Design review of the part built by this model. Coordinates are the model's own, in mm. A direction names the side the tool comes from. Coordinates: 2 decimals unless noted, no trailing zeros. Write each loop counter-clockwise with the first axis right and the second up, starting at its lowest first coordinate (ties: lowest second). Pieces come first, ordered by that corner, then holes.
Q1. For faces 1 (the cylindrical face through (-7.43, 0.76, 15.4)), 2 (the cylindrical face through (12.4, 0.76, 19.43)), list the 3-axis set-ups (+Z, -Z, +X, -X, +Y, -Y) from which the entire face can be reached by the end or side of a thin tool; tool diameter is ignored.
Q2. Take a section at A-A, the plane x = 0. Write out the cut boundary in (y, z), plus the area to 3 significant figures.
Q3. The part is to be moulded in two halves that separate along X. For faces 3 (the flat face through (-3, 1.5, -19)), 4 (the cylindrical face through (7.4, 0.76, 15.43)), 5 (the cylindrical face through (43.4, 0.74, -30.18)), say which applies: released by +X, released by -X, zero draft, split by the parting line, or undercut.
Q4. Take a section at C-C, the plane z = 15. Write out the cut boundary in (x, y).
Q5. Take a section at B-B, the plane x = 24.1. Write out the cut boundary in (y, z), plus the area to 3 significant figures.
Q6. Take a section at D-D, the plane y = 1. State how many separate pieces and enclosed holes the cut face has, plus the area to 3 significant figures.
Q7. For L1, parallel to X at y = 0.45, z = -27; L2, parallel to X at y = 0.65, z = 6.5; L3, parallel to Z at x = 38, y = 0.5, list the stretches that pass through material, from the lowest coordinate up.
Q8. For pin 1 Ø0.8 at (y, z) = (1, 13) entering from -X; pin 2 Ø0.8 at (x, y) = (-28, 0.5) entering from +Z; pin 3 Ø1.8 at (x, z) = (8, 18) entering from -Y, all flat-tipped, find the tip position at first contact; note any pin that passes through.
Autodesk Inventor part; units mm, degrees
ref_plane "YZ Plane" through (0, 0, 0) normal (1, 0, 0) x (0, 1, 0)
ref_plane "XZ Plane" through (0, 0, 0) normal (0, 1, 0) x (-1, 0, 0)
ref_plane "XY Plane" through (0, 0, 0) normal (0, 0, 1) x (1, 0, 0)
sketch "スケッチ1" plane through (0, 0, 0) normal (0, 1, 0) x (-1, 0, 0)
  line L0 (8, 18) -> (-8, 18) construction
  line L1 (-8, 18) -> (-8, -18) construction
  line L2 (-8, -18) -> (8, -18) construction
  line L3 (8, -18) -> (8, 18) construction
  line L4 (8, 18) -> (-8, -18) construction
  line L5 (-8, 18) -> (8, -18) construction
  circle A0 centre (8, -18) radius 1.1
  circle A1 centre (-8, -18) radius 1.1
  circle A2 centre (8, 18) radius 1.1
  circle A3 centre (-8, 18) radius 1.1
  line L6 (13, 20) -> (-13, 20)
  line L7 (-13, 20) -> (-13, -20)
  line L8 (-13, -20) -> (13, -20)
  line L9 (13, -20) -> (13, 20)
  line L10 (13, 20) -> (-13, -20) construction
  line L11 (-13, 20) -> (13, -20) construction
  line L12 (8, -10) -> (-8, -10)
  line L13 (-8, -10) -> (-8, 16)
  line L14 (-8, 16) -> (8, 16)
  line L15 (8, 16) -> (8, -10)
  circle A4 centre (0, -10) radius 8
  point P0 (0, 0)
  dimension "d0" = 2.2
  dimension "d1" = 16
  dimension "d2" = 36
  dimension "d5" = 16
  dimension "d8" = 36
  dimension "d11" = 2
  dimension "d12" = 5
  dimension "d15" = 2
  dimension "d16" = 10
extrude "押し出し1" add sketch "スケッチ1" along normal blind 1.5
fillet "フィレット1" radius 2 2 edges at (8, 0.75, 16) (-8, 0.75, 16)
sketch "スケッチ2" plane through (0, 1.5, 0) normal (0, 1, 0) x (1, 0, 0)
  line L0 (-44, -7.75) -> (44, -7.75)
  line L1 (44, -7.75) -> (44, 30.75)
  line L2 (44, 30.75) -> (-44, 30.75)
  line L3 (-44, 30.75) -> (-44, -7.75)
  line L4 (-44, -7.75) -> (44, 30.75) construction
  line L5 (44, -7.75) -> (-44, 30.75) construction
  line L6 (13, 20) -> (-13, 20)
  line L7 (-13, 20) -> (-13, -20)
  line L8 (-8, -14) -> (-8, 10)
  line L9 (8, 10) -> (8, -14)
  line L10 (13, -20) -> (13, 20)
  line L11 (13, 20) -> (-13, 20)
  line L12 (-13, 20) -> (-13, -20)
  line L13 (-13, -20) -> (13, -20)
  circle A0 centre (-8, -18) radius 1.1
  circle A1 centre (8, -18) radius 1.1
  circle A2 centre (8, 18) radius 1.1
  circle A3 centre (-8, 18) radius 1.1
  line L14 (-8, -14) -> (-8, 10)
  arc A4 (8, 10) -> (-8, 10) centre (0, 10) ccw
  line L15 (8, 10) -> (8, -14)
  arc A5 (6, -16) -> (8, -14) centre (6, -14) ccw
  line L16 (6, -16) -> (-6, -16)
  arc A6 (-8, -14) -> (-6, -16) centre (-6, -14) ccw
  line L17 (33, 26.75) -> (23, 26.75)
  line L18 (23, 26.75) -> (23, 29.75)
  line L19 (23, 29.75) -> (33, 29.75)
  line L20 (33, 29.75) -> (33, 26.75)
  circle A7 centre (38, 28.25) radius 1.1
  line L21 (28, 26.75) -> (28, 29.75) construction
  circle A8 centre (18, 28.25) radius 1.1
  line L22 (44, 11.5) -> (-44, 11.5) construction
  line L23 (33, -3.75) -> (23, -3.75)
  line L24 (23, -3.75) -> (23, -6.75)
  line L25 (23, -6.75) -> (33, -6.75)
  line L26 (33, -6.75) -> (33, -3.75)
  circle A9 centre (38, -5.25) radius 1.1
  line L27 (28, -3.75) -> (28, -6.75) construction
  circle A10 centre (18, -5.25) radius 1.1
  line L28 (0, 30.75) -> (0, -7.75) construction
  line L29 (-33, 26.75) -> (-23, 26.75)
  line L30 (-23, 26.75) -> (-23, 29.75)
  line L31 (-23, 29.75) -> (-33, 29.75)
  line L32 (-33, 29.75) -> (-33, 26.75)
  circle A11 centre (-38, 28.25) radius 1.1
  line L33 (-28, 26.75) -> (-28, 29.75) construction
  circle A12 centre (-18, 28.25) radius 1.1
  circle A13 centre (-18, -5.25) radius 1.1
  line L34 (-23, -3.75) -> (-23, -6.75)
  line L35 (-28, -3.75) -> (-28, -6.75) construction
  line L36 (-33, -3.75) -> (-23, -3.75)
  line L37 (-23, -6.75) -> (-33, -6.75)
  line L38 (-33, -6.75) -> (-33, -3.75)
  circle A14 centre (-38, -5.25) radius 1.1
  circle A15 centre (-31.9, -6.75) radius 1.1
  circle A16 centre (-24.1, -6.75) radius 1.1
  line L39 (-33, -5.25) -> (-28, -5.25) construction
  circle A17 centre (-31.9, -3.75) radius 1.1
  circle A18 centre (-24.1, -3.75) radius 1.1
  circle A19 centre (-31.9, 29.75) radius 1.1
  circle A20 centre (-24.1, 29.75) radius 1.1
  circle A21 centre (-31.9, 26.75) radius 1.1
  circle A22 centre (-24.1, 26.75) radius 1.1
  circle A23 centre (31.9, -6.75) radius 1.1
  circle A24 centre (24.1, -6.75) radius 1.1
  circle A25 centre (31.9, -3.75) radius 1.1
  circle A26 centre (24.1, -3.75) radius 1.1
  circle A27 centre (31.9, 29.75) radius 1.1
  circle A28 centre (31.9, 26.75) radius 1.1
  circle A29 centre (24.1, 26.75) radius 1.1
  circle A30 centre (24.1, 29.75) radius 1.1
  line L40 (33, 29.75) -> (33, 30.75)
  line L41 (23, 29.75) -> (23, 30.75)
  line L42 (-33, 29.75) -> (-33, 30.75)
  line L43 (-23, 29.75) -> (-23, 30.75)
  line L44 (33, -6.75) -> (33, -7.75)
  line L45 (23, -6.75) -> (23, -7.75)
  line L46 (-33, -6.75) -> (-33, -7.75)
  line L47 (-23, -6.75) -> (-23, -7.75)
  point P0 (0, 0)
  point P1 (0, 11.5)
  point P2 (-13, -7.75)
  point P3 (13, -7.75)
  point P4 (33, 28.25)
  point P5 (33, -5.25)
  point P6 (-13, 20)
  point P7 (-13, 20)
  point P8 (-33, 28.25)
  point P9 (33, -3.75)
  point P10 (33, -6.75)
  point P11 (30.8, -6.75)
  point P12 (25.2, -6.75)
  point P13 (23, -6.75)
  point P14 (23, -3.75)
  point P15 (23, -3.75)
  point P16 (-23, 29.75)
  point P17 (-23, 26.75)
  point P18 (-25.2, 26.75)
  point P19 (-30.8, 26.75)
  point P20 (-33, 26.75)
  point P21 (-33, 29.75)
  point P22 (-23, -3.75)
  point P23 (-23, -6.75)
  point P24 (-25.2, -6.75)
  point P25 (-30.8, -6.75)
  point P26 (-33, -3.75)
  point P27 (33, 29.75)
  point P28 (33, 26.75)
  point P29 (30.8, 26.75)
  point P30 (25.2, 26.75)
  point P31 (23, 26.75)
  point P32 (23, 29.75)
  point P33 (23, 29.75)
  point P34 (24.2, -6.75)
  point P35 (-29.8, 26.75)
  point P36 (24.2, 26.75)
  point P37 (27.2, -3.75)
  point P38 (23, -6.75)
  point P39 (30.8, -3.75)
  point P40 (-25.2, 29.75)
  point P41 (-32.8, 29.75)
  point P42 (27.2, 29.75)
  point P43 (30.8, 29.75)
  point P44 (23, 26.75)
  point P45 (-32.8, -3.75)
  point P46 (26.2, -3.75)
  point P47 (-31.8, 29.75)
  point P48 (-31.8, -3.75)
  point P49 (-25.2, -3.75)
  point P50 (26.2, 29.75)
  point P51 (25.2, -3.75)
  point P52 (-30.8, 29.75)
  point P53 (-30.8, -3.75)
  point P54 (25.2, 29.75)
  point P55 (32.3583, 30.75)
  point P56 (23.6417, 30.75)
  point P57 (-23.6417, 30.75)
  point P58 (-32.3583, 30.75)
  point P59 (-32.3583, -7.75)
  point P60 (-23.6417, -7.75)
  point P61 (23.6417, -7.75)
  point P62 (32.3583, -7.75)
  dimension "d30" = 2.2
  dimension "d19" = 31
  dimension "d22" = 10
  dimension "d23" = 3
  dimension "d25" = 2.2
  dimension "d26" = 5
  dimension "d27" = 6
  dimension "d29" = 1
  dimension "d31" = 18.25
extrude "押し出し3" add sketch "スケッチ2" against normal blind 1.5 contours L3 L2 L42 L32 A21 L29 A22 L30 L43 L41 L18 A29 L17 A28 L20 L40 L1 L0 L44 L26 A25 L23 A26 L24 L45 L10 L6 L7 L47 L34 A18 L36 A17 L38 L46
fillet "フィレット2" radius 2 8 edges at (44, 0.75, -30.75) (44, 0.75, 7.75) (13, 0.75, 7.75) (13, 0.75, 20) (-13, 0.75, 20) (-13, 0.75, 7.75) (-44, 0.75, 7.75) (-44, 0.75, -30.75)
sketch "スケッチ4" plane through (0, 1.5, 0) normal (0, 1, 0) x (1, 0, 0)
  line L0 (41, 23.65) -> (11, 23.65)
  line L1 (11, 23.65) -> (11, -0.65)
  line L2 (11, -0.65) -> (41, -0.65)
  line L3 (41, -0.65) -> (41, 23.65)
  arc A0 (30.8, 26.75) -> (33, 26.75) centre (31.9, 26.75) ccw
  line L4 (44, -5.75) -> (44, 28.75)
  arc A1 (33, -3.75) -> (30.8, -3.75) centre (31.9, -3.75) ccw
  line L5 (-11, -20) -> (11, -20) construction
  line L6 (0, -20) -> (0, 21) construction
  line L7 (-41, 23.65) -> (-11, 23.65)
  line L8 (-11, 23.65) -> (-11, -0.65)
  line L9 (-11, -0.65) -> (-41, -0.65)
  line L10 (-41, -0.65) -> (-41, 23.65)
  line L11 (-44, -5.75) -> (-44, 28.75)
  line L12 (11, -0.65) -> (41, 23.65) construction
  line L13 (44, 24.7931) -> (12.5888, -0.65)
  line L14 (39.4112, 23.65) -> (11, 0.6369)
  line L15 (-44, 24.7931) -> (-12.5888, -0.65)
  line L16 (-39.4112, 23.65) -> (-11, 0.6369)
  line L17 (8, 10) -> (8, -14)
  point P0 (0, 0)
  point P1 (31.9, 25.65)
  point P2 (41, 11.5)
  point P3 (31.9, -2.65)
  point P4 (-41, 11.5)
  point P5 (-15, 23)
  point P6 (41, 22.3631)
  point P7 (39.7412, 23.9172)
  point P8 (11.3299, 0.9041)
  point P9 (-11.3299, 0.9041)
  point P10 (17, 0.7731)
  point P11 (-12.5888, -0.65)
  point P12 (-41, 22.3631)
  point P13 (-39.4112, 23.65)
  point P14 (-17, 0.7731)
  dimension "d39" = 2
  dimension "d40" = 3
  dimension "d41" = 2
  dimension "d43" = 1
  dimension "d48" = 3
extrude "押し出し5" cut sketch "スケッチ4" against normal blind 1.5 contours L14 L1 L0 | L3 L2 L13 | L7 L8 L16 | L15 L9 L10
fillet "フィレット3" radius 2 12 edges at (-39.4112, 0.75, -23.65) (-41, 0.75, -22.3631) (-11, 0.75, -23.65) (-12.5888, 0.75, 0.65) (-41, 0.75, 0.65) (41, 0.75, 0.65) (39.4112, 0.75, -23.65) (41, 0.75, -22.3631) (11, 0.75, -23.65) (12.5888, 0.75, 0.65) (-11, 0.75, -0.6369) (11, 0.75, -0.6369)
equation "\"d5\" = d1"
equation "\"d8\" = d2"
properties part number "KSHI" material "アルミニウム 2014-T4"
Responses:
1. face 1: +Y, -Y
1. face 2: +Z, +X, +Y, -Y
2. outline: (0, -30.75) - (1.5, -30.75) - (1.5, -18) - (0, -18) - close; (0, 16) - (1.5, 16) - (1.5, 20) - (0, 20) - close
2. area: 25.1 mm2
3. face 3: zero draft
3. face 4: undercut
3. face 5: released by +X
4. outline: (-13, 0) - (-7.73, 0) - (-7.73, 1.5) - (-13, 1.5) - close; (7.73, 0) - (13, 0) - (13, 1.5) - (7.73, 1.5) - close
5. outline: (0, -25.65) - (1.5, -25.65) - (1.5, -23.65) - (0, -23.65) - close; (0, -11.25) - (1.5, -11.25) - (1.5, -8.67) - (0, -8.67) - close; (0, 0.65) - (1.5, 0.65) - (1.5, 2.65) - (0, 2.65) - close
5. area: 9.86 mm2
6. separate pieces: 1
6. enclosed holes: 17
6. area: 1,700 mm2
7. L1: x = -44 to -33, -23 to 23, 33 to 44
7. L2: x = -43.85 to -33, -23 to -8, 8 to 23, 33 to 43.85
7. L3: z = -30.75 to -29.35, -27.15 to -19.9, 0.65 to 4.15, 6.35 to 7.75
8. pin 1: stops at x = -13
8. pin 2: stops at z = 3.75
8. pin 3: passes through
